Autodesk Inventor part; units mm, degrees
ref_plane "YZ Plane" through (0, 0, 0) normal (1, 0, 0) x (0, 1, 0)
ref_plane "XZ Plane" through (0, 0, 0) normal (0, 1, 0) x (-1, 0, 0)
ref_plane "XY Plane" through (0, 0, 0) normal (0, 0, 1) x (1, 0, 0)
sketch "Sketch1" plane through (0, 0, 0) normal (0, 1, 0) x (-1, 0, 0)
  circle A0 centre (0, 0) radius 30 construction
  line L0 (64.9519, -37.5) -> (0, -75)
  line L1 (0, -75) -> (-64.9519, -37.5)
  line L2 (-64.9519, -37.5) -> (-64.9519, 37.5)
  line L3 (-64.9519, 37.5) -> (0, 75)
  line L4 (0, 75) -> (64.9519, 37.5)
  line L5 (64.9519, 37.5) -> (64.9519, -37.5)
  line L6 (58.5619, 31.7388) -> (52.2358, 31.7388)
  line L7 (52.2358, 31.7388) -> (52.2358, 12.78)
  line L8 (52.2358, 12.78) -> (58.5619, 12.78)
  line L9 (58.5619, 12.78) -> (58.5619, 31.7388)
  line L10 (64.9519, 0) -> (0, 0) construction
  line L11 (58.5619, -31.7388) -> (52.2358, -31.7388)
  line L12 (52.2358, -31.7388) -> (52.2358, -12.78)
  line L13 (52.2358, -12.78) -> (58.5619, -12.78)
  line L14 (58.5619, -12.78) -> (58.5619, -31.7388)
  line L15 (-40.3488, 44.3261) -> (-56.7676, 34.8467)
  line L16 (-56.7676, 34.8467) -> (-53.6045, 29.3681)
  line L17 (-53.6045, 29.3681) -> (-37.1857, 38.8475)
  line L18 (-37.1857, 38.8475) -> (-40.3488, 44.3261)
  line L19 (-15.0501, 51.6275) -> (-18.2131, 57.1061)
  line L20 (-18.2131, 57.1061) -> (-1.7943, 66.5855)
  line L21 (-1.7943, 66.5855) -> (1.3687, 61.1069)
  line L22 (1.3687, 61.1069) -> (-15.0501, 51.6275)
  line L23 (-18.2131, -57.1061) -> (-1.7943, -66.5855)
  line L24 (-1.7943, -66.5855) -> (1.3687, -61.1069)
  line L25 (1.3687, -61.1069) -> (-15.0501, -51.6275)
  line L26 (-15.0501, -51.6275) -> (-18.2131, -57.1061)
  line L27 (-37.1857, -38.8475) -> (-40.3488, -44.3261)
  line L28 (-40.3488, -44.3261) -> (-56.7676, -34.8467)
  line L29 (-56.7676, -34.8467) -> (-53.6045, -29.3681)
  line L30 (-53.6045, -29.3681) -> (-37.1857, -38.8475)
  dimension "d0" = 60
  dimension "d2" = 150
  dimension "d3" = 6.3261
  dimension "d4" = 18.9588
  dimension "d5" = 6.39
  dimension "d6" = 12.78
  dimension "d9" = 360
extrude "Extrusion1" add sketch "Sketch1" along normal blind 6.39
equation "\"d3\" = 0.99 * WoodThickness"
equation "\"d4\" = 0.25 * DiskGap"
equation "\"d5\" = WoodThickness"
equation "\"d6\" = 2 * WoodThickness"
equation "\"d11\" = WoodThickness"
properties part number "LightDiskTop" material "MDF Medium Density Fiberboard"
The listing builds one solid part. Answer for the finished solid, in the listing's coordinates (mm). A direction names the side the tool comes from. Give positions to 0.01 mm unless a question says otherwise; leave off trailing zeros. Write each loop counter-clockwise with the first axis right and the second up, starting at its lowest first coordinate (ties: lowest second). Pieces come first, ordered by that corner, then holes.
1) Section C-C (x = 47) is taken. Write down the section's boundary in (y, z), and give its area (3 significant figures).
2) For a pull along Z with two mould halves and no side action, classify faces 3 (the face through (-32.93, 3.15, -55.99)), 4 (the face through (55.21, 3.15, 32.15)), 5 (the face through (-58.562, 3, -22)), 6 (the face through (64.952, 3, -1)) as pulls with the +Z half, pulls with the -Z half, needs draft (parallel to the pull), parting line crosses it, or undercut.
3) Section D-D (x = -35) is taken. Write down the section's boundary in (y, z), and give its area (3 significant figures).
4) Find the intervals of material crossed by L1, parallel to X at y = 3.75, z = -24; L2, parallel to Z at x = 18, y = 0.75; L3, parallel to Z at x = -54, y = 2.75, in increasing order.
5) A tool of negligible diameter and unlimited length cuts with its end or side. For faces 1 (the face through (16.61, 3.15, 54.33)), 2 (the face through (1, 0, 1)), from which of +Z, -Z, +X, -X, +Y, -Y can it reach the whole face along a straight path? Write none if from no direction.
6) Given P1, Ø1, axis at y = 5.5, z = -53.5, coming from the -X side; P2, Ø1.5, axis at x = 43.5, y = 4, coming from the -Z side; P3, Ø1.9, axis at x = -54, y = 2, coming from the -Z side, each flat-ended and moving along its own axis, determine where each tip first touches the part or whether it passes through.
7) Section B-B (y = 2.75) is taken. Count the separate pieces of the cut face and the enclosed holes in it, and give its area (3 significant figures).
8) Section A-A (z = 17.5) is taken. Write down the section's boundary in (x, y).
Response:
1. outline: (0, -47.86) - (6.39, -47.86) - (6.39, -40.49) - (0, -40.49) - close; (0, -33.18) - (6.39, -33.18) - (6.39, 33.18) - (0, 33.18) - close; (0, 40.49) - (6.39, 40.49) - (6.39, 47.86) - (0, 47.86) - close
1. area: 518 mm2
2. face 3: pulls with the -Z half
2. face 4: undercut
2. face 5: undercut
2. face 6: needs draft
3. outline: (0, -54.79) - (6.39, -54.79) - (6.39, 54.79) - (0, 54.79) - close
3. area: 700 mm2
4. L1: x = -64.95 to -58.56, -52.24 to 64.95
4. L2: z = -64.61 to -57.23, -56.74 to 56.74, 57.23 to 64.61
4. L3: z = -43.82 to -31.74, -12.78 to 12.78, 31.74 to 43.82
5. face 1: +Y, -Y
5. face 2: +Z, -Z, +X, -X, -Y
6. P1: stops at x = -38.11
6. P2: stops at z = -50.32
6. P3: stops at z = -44.37
7. separate pieces: 1
7. enclosed holes: 6
7. area: 13,900 mm2
8. outline: (-64.95, 0) - (-58.56, 0) - (-58.56, 6.39) - (-64.95, 6.39) - close; (-52.24, 0) - (64.95, 0) - (64.95, 6.39) - (-52.24, 6.39) - close
